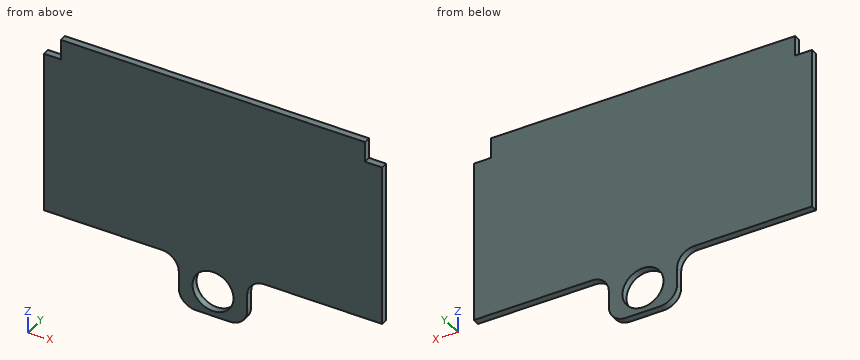
```python
from build123d import *

# Parameters (mm, degrees)
ESTRUSIONE_ESTRUSIONE1_DEPTH      = 48
ESTRUSIONE_ESTRUSIONE1_DEPTH_BACK = 6
SCHIZZO1_W                        = 89.03043591
SCHIZZO1_H                        = 2
SCHIZZO2_W                        = 45
SCHIZZO2_H                        = 2
ESTRUSIONE_ESTRUSIONE2_DEPTH      = 5
SCHIZZO3_W                        = 5
SCHIZZO3_H                        = 2
ESTRUSIONE_ESTRUSIONE3_DEPTH      = 3
SCHIZZO4_W                        = 20
SCHIZZO4_H                        = 15
ESTRUSIONE_ESTRUSIONE4_DEPTH      = 2
SCHIZZO5_R                        = 6
TAGLIO_ESTRUSIONE1_DEPTH          = 10
RACCORDO1_R                       = 5
CORPO_SPOSTA_COPIA3_START         = -88.5
CORPO_SPOSTA_COPIA3_OUTLINE_R     = 6
CORPO_SPOSTA_COPIA3_DEPTH         = 2
CORPO_SPOSTA_COPIA3_2_OUTLINE_R   = 6
CORPO_SPOSTA_COPIA3_2_DEPTH       = 2


# Read off the part's stored shape, not the designer's step: Corpo-Sposta/copia3
with BuildPart() as part:
    # Schizzo1 → Estrusione-Estrusione1 (new, two sides: drawn at the far end of the back side and taken through both)
    with BuildSketch(Plane.XY.offset(-ESTRUSIONE_ESTRUSIONE1_DEPTH_BACK)):
        with Locations((129.515217955, -87.5)):
            Rectangle(SCHIZZO1_W, SCHIZZO1_H)
    extrude(amount=ESTRUSIONE_ESTRUSIONE1_DEPTH + ESTRUSIONE_ESTRUSIONE1_DEPTH_BACK)

    # Schizzo2 → Estrusione-Estrusione2 (add)
    with BuildSketch(Plane(origin=(174.03043591, 0, 0), x_dir=(0, 0, -1), z_dir=(1, 0, 0))):
        with Locations((-22.5, -87.5)):
            Rectangle(SCHIZZO2_W, SCHIZZO2_H)
    estrusione_estrusione2 = extrude(amount=ESTRUSIONE_ESTRUSIONE2_DEPTH)

    # Schizzo3 → Estrusione-Estrusione3 (add)
    with BuildSketch(Plane.XY.offset(45)):
        with Locations((176.53043591, -87.5)):
            Rectangle(SCHIZZO3_W, SCHIZZO3_H)
    estrusione_estrusione3 = extrude(amount=ESTRUSIONE_ESTRUSIONE3_DEPTH)

    # Specchia1: Estrusione-Estrusione2, Estrusione-Estrusione3 across plane
    add(estrusione_estrusione2.mirror(Plane(origin=(129.515217955, 0, 0), x_dir=(0, 0, 1), z_dir=(1, 0, 0))))
    add(estrusione_estrusione3.mirror(Plane(origin=(129.515217955, 0, 0), x_dir=(0, 0, 1), z_dir=(1, 0, 0))))

    # Schizzo4 → Estrusione-Estrusione4 (add)
    with BuildSketch(Plane(origin=(0, -88.5, 0), x_dir=(-1, 0, 0), z_dir=(0, -1, 0))):
        with Locations((-129.515217955, -55.5)):
            Rectangle(SCHIZZO4_W, SCHIZZO4_H)
    extrude(amount=-ESTRUSIONE_ESTRUSIONE4_DEPTH)

    # Schizzo5 → Taglio-Estrusione1 (cut)
    with BuildSketch(Plane.XZ.offset(88.5)):
        with Locations(Location((129.515217955, 55.5, 0), (0, 0, 270))):
            Circle(SCHIZZO5_R)
    extrude(amount=-TAGLIO_ESTRUSIONE1_DEPTH, mode=Mode.SUBTRACT)

    # Raccordo1
    raccordo1_edges = [part.edges().sort_by_distance(p)[0] for p in [
        (139.515217955, -87.5, 63),
        (139.515217955, -87.5, 48),
        (119.515217955, -87.5, 48),
        (119.515217955, -87.5, 63),
    ]]
    fillet(raccordo1_edges, radius=RACCORDO1_R)

    # Corpo-Sposta/copia3 outline → Corpo-Sposta/copia3 (cut)
    with BuildSketch(Plane(origin=(0, 0, 0), x_dir=(1, 0, 0), z_dir=(0, 1, 0)).offset(CORPO_SPOSTA_COPIA3_START)):
        with BuildLine():
            Line((179.03043591, -48), (179.03043591, 0))
            Line((179.03043591, 0), (174.03043591, 0))
            Line((174.03043591, 0), (174.03043591, -6))
            Line((174.03043591, -6), (85, -6))
            Line((85, -6), (85, 0))
            Line((85, 0), (80, 0))
            Line((80, 0), (80, -48))
            Line((80, -48), (114.515217955, -48))
            ThreePointArc((114.515217955, -48), (118.050751861, -49.464466094), (119.515217955, -53))
            Line((119.515217955, -53), (119.515217955, -58))
            ThreePointArc((119.515217955, -58), (120.979684049, -61.535533906), (124.515217955, -63))
            Line((124.515217955, -63), (134.515217955, -63))
            ThreePointArc((134.515217955, -63), (138.050751861, -61.535533906), (139.515217955, -58))
            Line((139.515217955, -58), (139.515217955, -53))
            ThreePointArc((139.515217955, -53), (140.979684049, -49.464466094), (144.515217955, -48))
            Line((144.515217955, -48), (179.03043591, -48))
        make_face()
        with Locations((129.515217955, -55.5)):
            Circle(CORPO_SPOSTA_COPIA3_OUTLINE_R, mode=Mode.SUBTRACT)
    extrude(amount=CORPO_SPOSTA_COPIA3_DEPTH, mode=Mode.SUBTRACT)

    # Corpo-Sposta_copia3 2 outline → Corpo-Sposta_copia3 2 (add)
    with BuildSketch(Plane(origin=(0, 0, 0), x_dir=(1, 0, 0), z_dir=(0, 1, 0)).offset(CORPO_SPOSTA_COPIA3_START)):
        with BuildLine():
            Line((179.03043591, 0), (179.03043591, 48))
            Line((179.03043591, 48), (144.515217955, 48))
            ThreePointArc((144.515217955, 48), (140.979684049, 49.464466094), (139.515217955, 53))
            Line((139.515217955, 53), (139.515217955, 58))
            ThreePointArc((139.515217955, 58), (138.050751861, 61.535533906), (134.515217955, 63))
            Line((134.515217955, 63), (124.515217955, 63))
            ThreePointArc((124.515217955, 63), (120.979684049, 61.535533906), (119.515217955, 58))
            Line((119.515217955, 58), (119.515217955, 53))
            ThreePointArc((119.515217955, 53), (118.050751861, 49.464466094), (114.515217955, 48))
            Line((114.515217955, 48), (80, 48))
            Line((80, 48), (80, 0))
            Line((80, 0), (85, 0))
            Line((85, 0), (85, 6))
            Line((85, 6), (174.03043591, 6))
            Line((174.03043591, 6), (174.03043591, 0))
            Line((174.03043591, 0), (179.03043591, 0))
        make_face()
        with Locations((129.515217955, 55.5)):
            Circle(CORPO_SPOSTA_COPIA3_2_OUTLINE_R, mode=Mode.SUBTRACT)
    extrude(amount=CORPO_SPOSTA_COPIA3_2_DEPTH)


solid = part.part
```
Build history of the part. All positions in model axes, mm. Round coordinates to 2 decimals unless told otherwise and drop trailing zeros. Write each loop counter-clockwise with the first axis right and the second up, starting at its lowest first coordinate (ties: lowest second). Pieces come first, ordered by that corner, then holes. Notation, with made-up numbers: (18.25, -8) -> (43.25, -8) arc R26 ccw to (43.25, 31) -> close; hole circle Ø7 at (80, 85). An arc over 180 degrees is marked (long way). Put each result on its own line as item: value.
Item 1: Slice it at A-A, the plane z = -55.5. Give the cut face in (x, y), plus the area to 3 significant figures.
Here are the results:
outline: (119.52, -88.5) -> (123.52, -88.5) -> (123.52, -86.5) -> (119.52, -86.5) -> close; (135.52, -88.5) -> (139.52, -88.5) -> (139.52, -86.5) -> (135.52, -86.5) -> close
area: 16.0 mm^2
Item 2: Slice it at D-D, the plane z = 1.5. Give the cut face in (x, y).
Here are the results:
outline: (85, -88.5) -> (174.03, -88.5) -> (174.03, -86.5) -> (85, -86.5) -> close
Item 3: Wall check: probe 1 along X at (y, z) = (-87.9, -55.5); probe 2 along Z at (x, y) = (129, -88); probe 3 along Z at (x, y) = (107, -87.85). Give the ranges that are in metal, low to high. Write a range as from..to.
Here are the results:
probe 1: x = 119.52..123.52, 135.52..139.52
probe 2: z = -63..-61.48, -49.52..6
probe 3: z = -48..6
Item 4: Slice it at C-C, the plane x = 111. Give the cut face in (y, z).
Here are the results:
outline: (-88.5, -48) -> (-86.5, -48) -> (-86.5, 6) -> (-88.5, 6) -> close
Item 5: Slice it at B-B, the plane y = -87.95. Give the cut face in (x, z).
Here are the results:
outline: (80, -48) -> (114.52, -48) arc R5 cw to (119.52, -53) -> (119.52, -58) arc R5 ccw to (124.52, -63) -> (134.52, -63) arc R5 ccw to (139.52, -58) -> (139.52, -53) arc R5 cw to (144.52, -48) -> (179.03, -48) -> (179.03, 0) -> (174.03, 0) -> (174.03, 6) -> (85, 6) -> (85, 0) -> (80, 0) -> close; hole circle Ø12 at (129.52, -55.5)
Item 6: Flat gauge pins, fed straight in: P1, Ø1, axis at x = 82, y = -87, coming from the +Z side; P2, Ø0.6, axis at y = -87.5, z = 4, coming from the +X side; P3, Ø0.6, axis at x = 169.5, y = -87.5, coming from the -Z side; P4, Ø7, axis at x = 129.52, z = -55.5, coming from the +Y side (3 decimals). Where does each tip first touch, or does it go through?
Here are the results:
P1: stops at z = 0
P2: stops at x = 174.03
P3: stops at z = -48
P4: passes through
